from build123d import *

# Parameters (mm, degrees)
F0_W     = 60
F0_H     = 60
F1_DEPTH = 82
F2_SIZE  = 10
F3_W     = 12.7
F3_H     = 12.7
F4_DEPTH = 12.7
F5_W     = 12.7
F5_H     = 12.7
F6_DEPTH = 12.7


with BuildPart() as f1:
    # F0 (on Top) → F1 (new body)
    with BuildSketch(Plane.XY):
        Rectangle(F0_W, F0_H)
    extrude(amount=F1_DEPTH)

    # F2
    f2_edges = [f1.edges().sort_by_distance(p)[0] for p in [
        (30, -30, 41),
        (30, 30, 41),
        (-30, -30, 41),
        (-30, 30, 41),
    ]]
    chamfer(f2_edges, length=F2_SIZE)

    # F3 (on face) → F4 (cut)
    with BuildSketch(Plane.XY.offset(82)):
        Rectangle(F3_W, F3_H)
    extrude(amount=-F4_DEPTH, mode=Mode.SUBTRACT)

    # F5 (on face) → F6 (join)
    with BuildSketch(Plane(origin=(0, 0, 0), x_dir=(1, 0, 0), z_dir=(0, 0, -1))):
        Rectangle(F5_W, F5_H)
    extrude(amount=F6_DEPTH)


solid = f1.part
Can you work these out from the model? Positions are in its coordinate system, mm. A direction names the side the tool comes from. Round coordinates to 2 decimals unless told otherwise and drop trailing zeros. Write each loop counter-clockwise with the first axis right and the second up, starting at its lowest first coordinate (ties: lowest second). Pieces come first, ordered by that corner, then holes. Notation, with made-up numbers: (-7.5, 84) -> (46.5, 84) arc R14 cw to (46.5, 109) -> close; hole circle Ø5 at (56, -3). An arc over 180 degrees is marked (long way). One line per question, with ' | ' between items. Start each with the question number.
1) On a 3-axis mill with a long thin cutter (end or side, diameter ignored), from which of +Z, -Z, +X, -X, +Y, -Y can I reach the whole of each face in a straight line? I mean faces 4 (the flat face through (25, 25, 40)), 5 (the flat face through (0, 30, 40)), 6 (the flat face through (6.35, 0, -6)), 7 (the flat face through (0, 6.35, 76)), 8 (the flat face through (-6.35, 0, -6)). Say none if no direction works.
2) I'm going to push flat-ended pins straight in: P1, Ø4, axis at x = -1, z = -6, coming from the +Y side; P2, Ø4, axis at y = -23, z = 19.5, coming from the +X side; P3, Ø4, axis at y = 2, z = -3.5, coming from the -X side. Where does each tip first touch, or does it pass through?
3) Suppose I cut it at B-B on x = -18.5. Write out the boundary of the cut face in (y, z).
4) I need wall thicknesses on line 1 (X direction, y = -4, z = 71); line 2 (Z direction, x = -22.5, y = -19.5); line 3 (Y direction, x = 21, z = 16). Which ranges of each line are inside material? Lowest first, please. Write a range as [from, to].
5) Suppose I cut it at A-A on z = 33. Write out the boundary of the cut face in (x, y), then the cut area to 3 significant figures.
6) If we mould it in two halves opening along Y, with no side actions, what happens to faces 1 (the flat face through (0, -6.35, -6)), 2 (the flat face through (0, 0, 69.3)), 3 (the flat face through (0, 6.35, -6))? For each: released by +Y, released by -Y, zero draft, split by the parting line, or undercut.
Return value:
1) face 4: +Z, -Z, +X, +Y | face 5: +Z, -Z, +X, -X, +Y | face 6: -Z, +X, +Y, -Y | face 7: +Z | face 8: -Z, -X, +Y, -Y
2) P1: stops at y = 6.35 | P2: stops at x = 29 | P3: stops at x = -6.35
3) outline: (-30, 0) -> (30, 0) -> (30, 82) -> (-30, 82) -> close
4) line 1: x = [-30, -6.35], [6.35, 30] | line 2: z = [0, 82] | line 3: y = [-29, 29]
5) outline: (-30, -20) -> (-20, -30) -> (20, -30) -> (30, -20) -> (30, 20) -> (20, 30) -> (-20, 30) -> (-30, 20) -> close | area: 3,400 mm2
6) face 1: released by -Y | face 2: undercut | face 3: released by +Y
